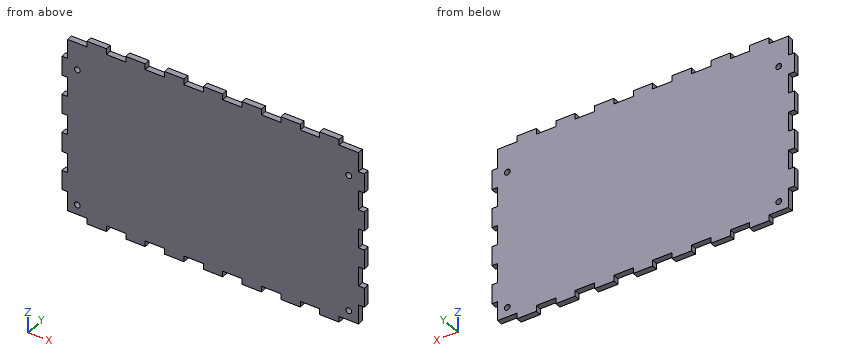
from build123d import *

# Parameters (mm, degrees)
BOSS_EXTRUDE1_DEPTH = 3
SKETCH2_R           = 1.5
CUT_EXTRUDE1_DEPTH  = 3


with BuildPart() as part:
    # Sketch1 → Boss-Extrude1 (new body)
    with BuildSketch(Plane(origin=(0, 0, 0), x_dir=(1, 0, 0), z_dir=(0, 1, 0))):
        Polygon((-5, 48), (5, 48), (5, 45), (15, 45), (15, 48), (25, 48), (25, 45), (35, 45), (35, 48), (45, 48), (45, 45), (55, 45), (55, 48), (65, 48), (65, 45), (75, 45), (75, 35), (78, 35), (78, 25), (75, 25), (75, 15), (78, 15), (78, 5), (75, 5), (75, -5), (78, -5), (78, -15), (75, -15), (75, -25), (78, -25), (78, -35), (75, -35), (75, -45), (65, -45), (65, -48), (55, -48), (55, -45), (45, -45), (45, -48), (35, -48), (35, -45), (25, -45), (25, -48), (15, -48), (15, -45), (5, -45), (5, -48), (-5, -48), (-5, -45), (-15, -45), (-15, -48), (-25, -48), (-25, -45), (-35, -45), (-35, -48), (-45, -48), (-45, -45), (-55, -45), (-55, -48), (-65, -48), (-65, -45), (-75, -45), (-75, -35), (-78, -35), (-78, -25), (-75, -25), (-75, -15), (-78, -15), (-78, -5), (-75, -5), (-75, 5), (-78, 5), (-78, 15), (-75, 15), (-75, 25), (-78, 25), (-78, 35), (-75, 35), (-75, 45), (-65, 45), (-65, 48), (-55, 48), (-55, 45), (-45, 45), (-45, 48), (-35, 48), (-35, 45), (-25, 45), (-25, 48), (-15, 48), (-15, 45), (-5, 45), align=None)
    extrude(amount=BOSS_EXTRUDE1_DEPTH)

    # Sketch2 → Cut-Extrude1 (cut)
    with BuildSketch(Plane(origin=(0, 3, 0), x_dir=(1, 0, 0), z_dir=(0, 1, 0))):
        with Locations(Location((70, 40, 0), (0, 0, 270))):
            Circle(SKETCH2_R)
        with Locations(Location((70, -31, 0), (0, 0, 270))):
            Circle(SKETCH2_R)
        with Locations(Location((-70, 40, 0), (0, 0, 90))):
            Circle(SKETCH2_R)
        with Locations(Location((-70, -31, 0), (0, 0, 90))):
            Circle(SKETCH2_R)
    extrude(amount=-CUT_EXTRUDE1_DEPTH, mode=Mode.SUBTRACT)


solid = part.part
Model file for the job. Use its own axes, mm. Give positions to 0.01 mm unless a question says otherwise; leave off trailing zeros. Order: outer loops, then holes, each group sorted by start corner. A loop starts at its lowest first (then second) coordinate and runs counter-clockwise, first axis right, second up. Notation, with made-up numbers: M 80,9 L 114,9 A7 ccw 114,19 Z; hole C 67,-31 d10. An arc over 180 degrees is marked long. Write item = value, one per line.
Q1. Flat gauge pins, fed straight in: pin 1 (1.5 mm diameter, centred on x = 76.5, y = 2, fed in from +Z); pin 2 (1.5 mm diameter, centred on x = -71, y = 1.5, fed in from -Z); pin 3 (1.5 mm diameter, centred on y = 1.5, z = -46, fed in from +X); pin 4 (3 mm diameter, centred on x = -34.5, z = 5, fed in from -Y). Where does each tip first touch, or does it go through?
Derived:
pin_1 = 35
pin_2 = -45
pin_3 = 65
pin_4 = 0
Q2. Cut at D-D, the plane x = 29. List the corners of the cut face in (y, z), then the cut area to 3 significant figures.
Derived:
outline = M 0,-45 L 3,-45 L 3,45 L 0,45 Z
area = 270 mm2
Q3. Cut at B-B, the plane x = -70. List the corners of the cut face in (y, z), then the cut area to 3 significant figures.
Derived:
outline = M 0,-45 L 3,-45 L 3,-41.5 L 0,-41.5 Z; M 0,-38.5 L 3,-38.5 L 3,29.5 L 0,29.5 Z; M 0,32.5 L 3,32.5 L 3,45 L 0,45 Z
area = 252 mm2
Q4. Cut at A-A, the plane z = 31. List the corners of the cut face in (x, y), then the cut area to 3 significant figures.
Derived:
outline = M -78,0 L -71.5,0 L -71.5,3 L -78,3 Z; M -68.5,0 L 68.5,0 L 68.5,3 L -68.5,3 Z; M 71.5,0 L 78,0 L 78,3 L 71.5,3 Z
area = 450 mm2
Q5. Drill centre lines: line 1 (Z direction, x = -70, y = 0.75); line 2 (X direction, y = 1.4, z = 31); line 3 (X direction, y = 1.65, z = -40). Where is each one in solid material? Low to high. Write a range as [from, to].
Derived:
line_1 = [-45, -41.5], [-38.5, 29.5], [32.5, 45]
line_2 = [-78, -71.5], [-68.5, 68.5], [71.5, 78]
line_3 = [-75, -71.5], [-68.5, 68.5], [71.5, 75]
Q6. Cut at C-C, the plane y = 2.45. Count the separate pieces of the cut face and the enclosed holes in it, then the cut area to 3 significant figures.
Derived:
separate_pieces = 1
enclosed_holes = 4
area = 14,100 mm2
